Job drawing, mm, ordinate dimensions from the low corner. One solid piece. A direction names the side the tool comes from. Coordinates: 2 decimals unless noted, no trailing zeros. Write each loop counter-clockwise with the first axis right and the second up, starting at its lowest first coordinate (ties: lowest second). Pieces come first, ordered by that corner, then holes. Notation, with made-up numbers: (34.5, -33.5) -> (71.5, -33.5) arc R12 cw to (71.5, -12.5) -> close; hole circle Ø9 at (-3, 57.25). An arc over 180 degrees is marked (long way). Answer as a JSON object with one key per item and string values. Group by question number.
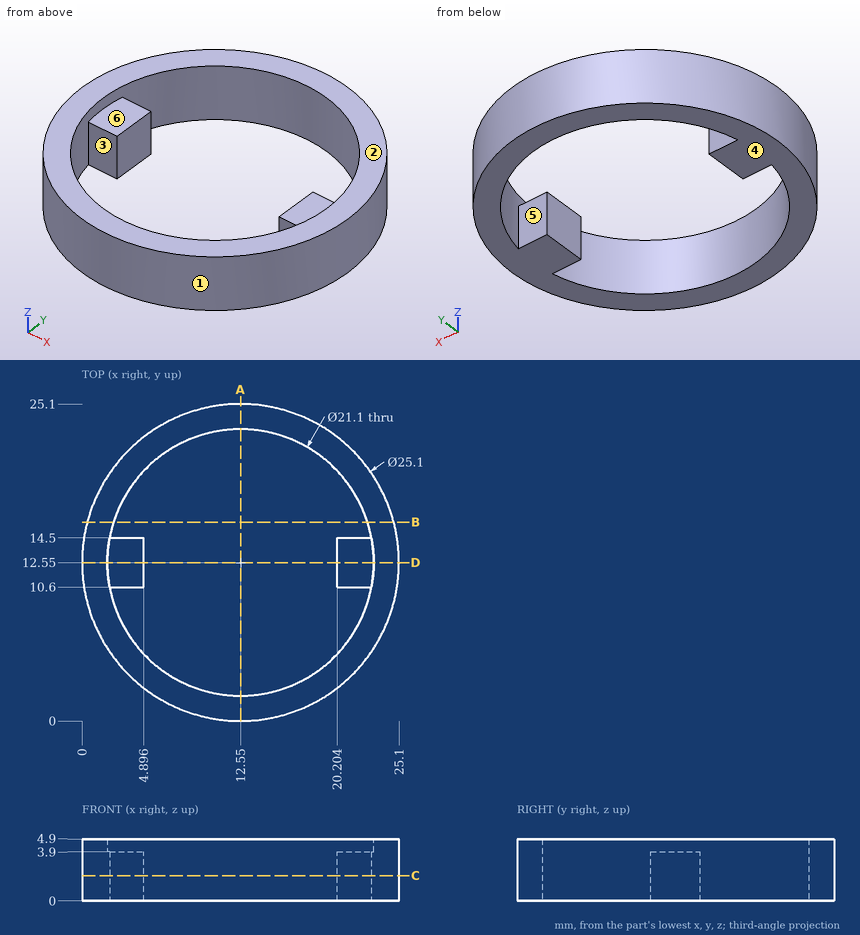
(1) 3-axis set-ups, long thin cutter, end or side, ignore diameter. For the marked faces 4, 5 and 6: which of +Z, -Z, +X, -X, +Y, -Y reach the whole face in a straight line?
(2) Pull direction Y, two halves, no side cores. Call the marked faces 1, 2 and 3: released by +Y, released by -Y, zero draft, split by the parting line, or undercut.
(3) Cut at A-A on x = 12.55. List the corners of the cut face in (y, z), plus the area to 3 significant figures.
(4) Cut at D-D on y = 12.55. List the corners of the cut face in (x, z), plus the area to 3 significant figures.
(5) Wall check: probe 1 along Y at (x, z) = (12.55, 1.35); probe 2 along X at (y, z) = (6, 2.15) (1 decimal). Give the ranges that are in metal, low to high.
(6) Cut at C-C on z = 2. List the corners of the cut face in (x, y).
(7) Cut at B-B on y = 15.75. List the corners of the cut face in (x, z) (1 decimal).
(8) Pin check, flat tips, straight feed: pin 1 (2 mm diameter, centred on x = 3, z = 1, fed in from -Y); pin 2 (3 mm diameter, centred on x = 4, y = 11.5, fed in from +Z); pin 3 (1.5 mm diameter, centred on x = 4.5, z = 3, fed in from -Y); pin 4 (12.5 mm diameter, centred on x = 12.55, y = 12.55, fed in from +Z). Stop position of each tip, or through.
Results found:
{
 "1": {"face 4": "-Z, +X, -X, +Y, -Y", "face 5": "+Z, -Z", "face 6": "+Z"},
 "2": {"face 1": "split by the parting line", "face 2": "zero draft", "face 3": "undercut"},
 "3": {"outline": "(0, 0) -> (2, 0) -> (2, 4.9) -> (0, 4.9) -> close; (23.1, 0) -> (25.1, 0) -> (25.1, 4.9) -> (23.1, 4.9) -> close", "area": "19.6 mm²"},
 "4": {"outline": "(0, 0) -> (4.9, 0) -> (4.9, 3.9) -> (2, 3.9) -> (2, 4.9) -> (0, 4.9) -> close; (20.2, 0) -> (25.1, 0) -> (25.1, 4.9) -> (23.1, 4.9) -> (23.1, 3.9) -> (20.2, 3.9) -> close", "area": "42.2 mm²"},
 "5": {"probe 1": "y = 0 to 2, 23.1 to 25.1", "probe 2": "x = 1.8 to 4.3, 20.8 to 23.3"},
 "6": {"outline": "circle Ø25.1 at (12.55, 12.55); hole (2.18, 10.6) arc R10.55 ccw to (22.92, 10.6) -> (20.2, 10.6) -> (20.2, 14.5) -> (22.92, 14.5) arc R10.55 ccw to (2.18, 14.5) -> (4.9, 14.5) -> (4.9, 10.6) -> close"},
 "7": {"outline": "(0.4, 0) -> (2.5, 0) -> (2.5, 4.9) -> (0.4, 4.9) -> close; (22.6, 0) -> (24.7, 0) -> (24.7, 4.9) -> (22.6, 4.9) -> close"},
 "8": {"pin 1": "stops at y = 3.36", "pin 2": "stops at z = 3.9", "pin 3": "stops at y = 2.34", "pin 4": "passes through"}
}
